```python
from build123d import *

# Parameters (mm, degrees)
CROQUIS1_W                = 5
CROQUIS1_H                = 5
SALIENTE_EXTRUIR1_DEPTH   = 41
SALIENTE_EXTRUIR1_2_DEPTH = 41
SALIENTE_EXTRUIR1_3_DEPTH = 41
SALIENTE_EXTRUIR1_4_DEPTH = 41
CROQUIS2_W                = 42
CROQUIS2_H                = 51
SALIENTE_EXTRUIR2_DEPTH   = 5
CROQUIS3_R                = 0.79375
CORTAR_EXTRUIR1_DEPTH     = 41


with BuildPart() as part:
    # Croquis1 → Saliente-Extruir1 (new body)
    with BuildSketch(Plane(origin=(0, 0, 0), x_dir=(1, 0, 0), z_dir=(0, 1, 0))):
        with Locations((-18.565940407, 9.143956682)):
            Rectangle(CROQUIS1_W, CROQUIS1_H)
    extrude(amount=SALIENTE_EXTRUIR1_DEPTH)



with BuildPart() as body_2:
    # Croquis1 → Saliente-Extruir1 2 (new body)
    with BuildSketch(Plane(origin=(0, 0, 0), x_dir=(1, 0, 0), z_dir=(0, 1, 0))):
        with Locations((18.434059593, 9.143956682)):
            Rectangle(CROQUIS1_W, CROQUIS1_H)
    extrude(amount=SALIENTE_EXTRUIR1_2_DEPTH)


with BuildPart() as body_3:
    # Croquis1 → Saliente-Extruir1 3 (new body)
    with BuildSketch(Plane(origin=(0, 0, 0), x_dir=(1, 0, 0), z_dir=(0, 1, 0))):
        with Locations((-18.565940407, -36.856043318)):
            Rectangle(CROQUIS1_W, CROQUIS1_H)
    extrude(amount=SALIENTE_EXTRUIR1_3_DEPTH)


with BuildPart() as body_4:
    # Croquis1 → Saliente-Extruir1 4 (new body)
    with BuildSketch(Plane(origin=(0, 0, 0), x_dir=(1, 0, 0), z_dir=(0, 1, 0))):
        with Locations((18.434059593, -36.856043318)):
            Rectangle(CROQUIS1_W, CROQUIS1_H)
    extrude(amount=SALIENTE_EXTRUIR1_4_DEPTH)


with BuildPart() as part_1:
    add(part.part)

    add(body_2.part)  # Saliente-Extruir2 merges body 2

    add(body_3.part)  # Saliente-Extruir2 merges body 3

    add(body_4.part)  # Saliente-Extruir2 merges body 4
    # Croquis2 → Saliente-Extruir2 (add)
    with BuildSketch(Plane(origin=(0, 0, 0), x_dir=(1, 0, 0), z_dir=(0, 1, 0))):
        with Locations((-0.065940407, -13.856043318)):
            Rectangle(CROQUIS2_W, CROQUIS2_H)
    extrude(amount=SALIENTE_EXTRUIR2_DEPTH)

    # Croquis3 → Cortar-Extruir1 (cut)
    with BuildSketch(Plane(origin=(0, 41, 0), x_dir=(1, 0, 0), z_dir=(0, 1, 0))):
        with Locations(Location((-18.565940407, 9.143956682, 0), (0, 0, 270))):
            Circle(CROQUIS3_R)
        with Locations(Location((-18.565940407, -36.856043318, 0), (0, 0, 270))):
            Circle(CROQUIS3_R)
    cortar_extruir1 = extrude(amount=-CORTAR_EXTRUIR1_DEPTH, mode=Mode.SUBTRACT)

    # Simetría1: Cortar-Extruir1 across plane
    add(cortar_extruir1.mirror(Plane(origin=(0, 0, 0), x_dir=(0, 0, 1), z_dir=(1, 0, 0))), mode=Mode.SUBTRACT)


solid = part_1.part
```
Check sheet for the modelled part. Datum: model origin and axes. Units: mm. A direction names the side the tool comes from. Round coordinates to 2 decimals unless told otherwise and drop trailing zeros. Loops run counter-clockwise (first coordinate to the right, second up) from the corner with the lowest first, then second, coordinate; pieces in that order, holes last. Notation, with made-up numbers: (59, 41) -> (117, 41) arc R25 cw to (117, 62) -> close; hole circle Ø9 at (-9.75, -40). An arc over 180 degrees is marked (long way). Write item = value, one per line. Start each with the question number.
1) Sectioned sample at A-A, the plane y = 8. Record the cut outline in (x, z).
2) Gauge pin test, flat ends, axial feed: pin 1 Ø1.3 at (x, z) = (18.57, 36.86) entering from -Y; pin 2 Ø1.5 at (x, z) = (4, 34) entering from +Y. Record the tip position at first contact, or that the pin passes through.
3) Set-up check for faces 4 (the flat face through (-16.066, 23, 37)), 5 (the flat face through (18, 23, 34.356)), 6 (the flat face through (18, 41, 36)): record each of +Z, -Z, +X, -X, +Y, -Y from which the full face is reachable in a straight line by a thin tool's end or side.
4) Release check for a two-part mould opening along Z. For faces 1 (the flat face through (15.934, 23, -9)), 2 (the flat face through (18, 23, -6.644)), 3 (the flat face through (-2, 4, 39.356)) record: released by +Z, released by -Z, zero draft, split by the parting line, or undercut.
5) Thickness scan on probe 1 along X at (y, z) = (3, 37); probe 2 along X at (y, z) = (12.5, -9); probe 3 along Z at (x, y) = (16, 10). Record the ranges inside material, lowest first.
6) Sectioned sample at C-C, the plane x = 15. Record the cut outline in (y, z).
7) Sectioned sample at B-B, the plane z = 5.5. Record the cut outline in (x, y).
Results are:
q1.outline = (-21.07, -11.64) -> (-16.07, -11.64) -> (-16.07, -6.64) -> (-21.07, -6.64) -> close; (-21.07, 34.36) -> (-16.07, 34.36) -> (-16.07, 39.36) -> (-21.07, 39.36) -> close; (15.93, -11.64) -> (20.93, -11.64) -> (20.93, -6.64) -> (15.93, -6.64) -> close; (15.93, 34.36) -> (20.93, 34.36) -> (20.93, 39.36) -> (15.93, 39.36) -> close; hole circle Ø1.59 at (-18.57, -9.14); hole circle Ø1.59 at (-18.57, 36.86); hole circle Ø1.59 at (18.57, -9.14); hole circle Ø1.59 at (18.57, 36.86)
q2.pin_1 = through
q2.pin_2 = 5
q3.face_4 = +Z, -Z, +Y
q3.face_5 = +X, -X, +Y
q3.face_6 = +Z, -Z, +X, -X, +Y
q4.face_1 = zero draft
q4.face_2 = undercut
q4.face_3 = released by +Z
q5.probe_1 = -21.07 to -19.35, -17.79 to 17.79, 19.35 to 20.93
q5.probe_2 = -21.07 to -19.35, -17.79 to -16.07, 15.93 to 17.79, 19.35 to 20.93
q5.probe_3 = -11.64 to -6.64, 34.36 to 39.36
q6.outline = (0, -11.64) -> (5, -11.64) -> (5, 39.36) -> (0, 39.36) -> close
q7.outline = (-21.07, 0) -> (20.93, 0) -> (20.93, 5) -> (-21.07, 5) -> close
